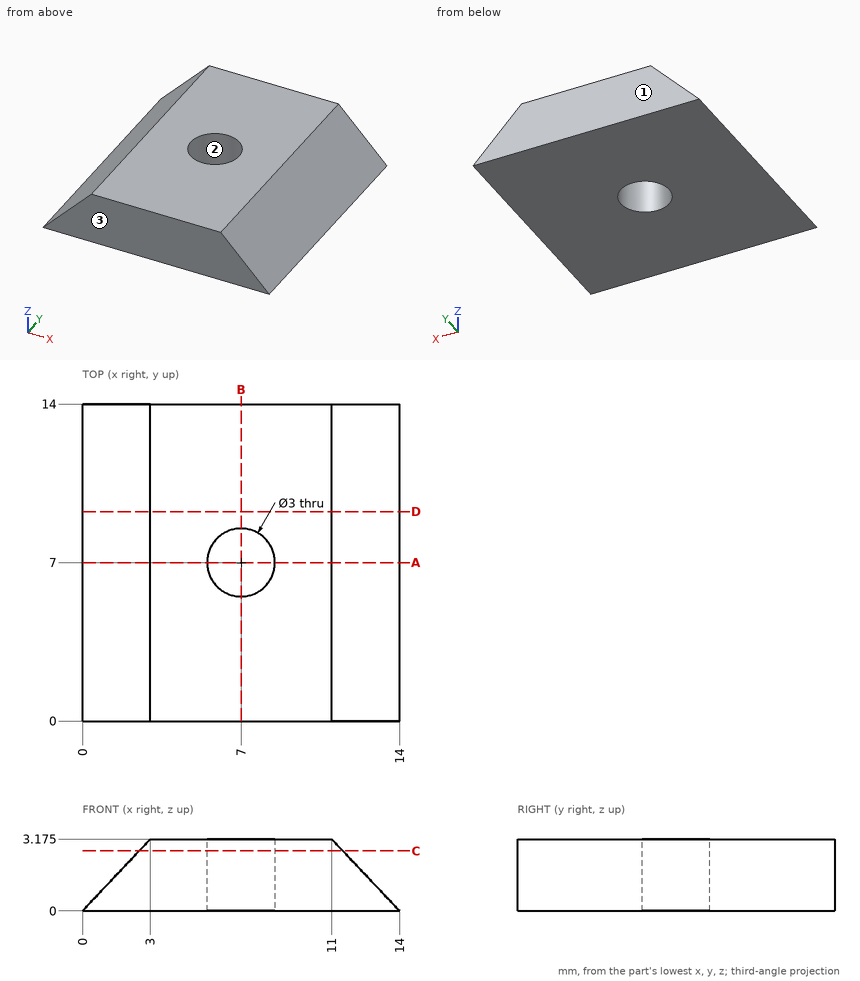
Verification items for this drawing (mm, ordinates from the low corner). Give positions to 0.01 mm unless a question says otherwise; leave off trailing zeros. Loops run counter-clockwise (first coordinate to the right, second up) from the corner with the lowest first, then second, coordinate; pieces in that order, holes last. Notation, with made-up numbers: M -6,44 L 7,44 A22 ccw 7,73 Z; hole C 50.25,30.25 d2. An arc over 180 degrees is marked long. Answer in a Markdown table with one row per item.
1) Depth check by flat-ended pin: pin 1 (2.5 mm diameter, centred on x = 7, y = 7, fed in from +Z). Enter the tip coordinate at first touch or a pass-through.
Solutions:
| item | result |
|---|---|
| pin 1 | passes through |
2) Cross-section at C-C (z = 2.65). Enter the section's corners in (x, y).
Solutions:
| item | result |
|---|---|
| outline | M 2.5,0 L 11.5,0 L 11.5,14 L 2.5,14 Z; hole C 7,7 d3 |
3) Thickness scan on line 1 (Y direction, x = 7, z = 1.7); line 2 (X direction, y = 6.75, z = 2); line 3 (X direction, y = 8.25, z = 1.2). Record the ranges inside material, lowest first.
Solutions:
| item | result |
|---|---|
| line 1 | y = 0 to 5.5, 8.5 to 14 |
| line 2 | x = 1.89 to 5.52, 8.48 to 12.11 |
| line 3 | x = 1.13 to 6.17, 7.83 to 12.87 |
4) Cross-section at D-D (y = 9.25). Enter the section's corners in (x, z) (3 decimals), plus the area to 3 significant figures.
Solutions:
| item | result |
|---|---|
| outline | M 0,0 L 14,0 L 11,3.175 L 3,3.175 Z |
| area | 34.9 mm^2 |
5) Cross-section at A-A (y = 7). Enter the section's corners in (x, z) (3 decimals), plus the area to 3 significant figures.
Solutions:
| item | result |
|---|---|
| outline | M 0,0 L 5.5,0 L 5.5,3.175 L 3,3.175 Z; M 8.5,0 L 14,0 L 11,3.175 L 8.5,3.175 Z |
| area | 25.4 mm^2 |
6) Mould release check, pull along Y, two halves, no side actions. Record for the marked faces 1, 2 and 3: released by +Y, released by -Y, zero draft, split by the parting line, or undercut.
Solutions:
| item | result |
|---|---|
| face 1 | released by +Y |
| face 2 | undercut |
| face 3 | released by -Y |
7) Cross-section at B-B (x = 7). Enter the section's corners in (y, z) (3 decimals).
Solutions:
| item | result |
|---|---|
| outline | M 0,0 L 5.5,0 L 5.5,3.175 L 0,3.175 Z; M 8.5,0 L 14,0 L 14,3.175 L 8.5,3.175 Z |
